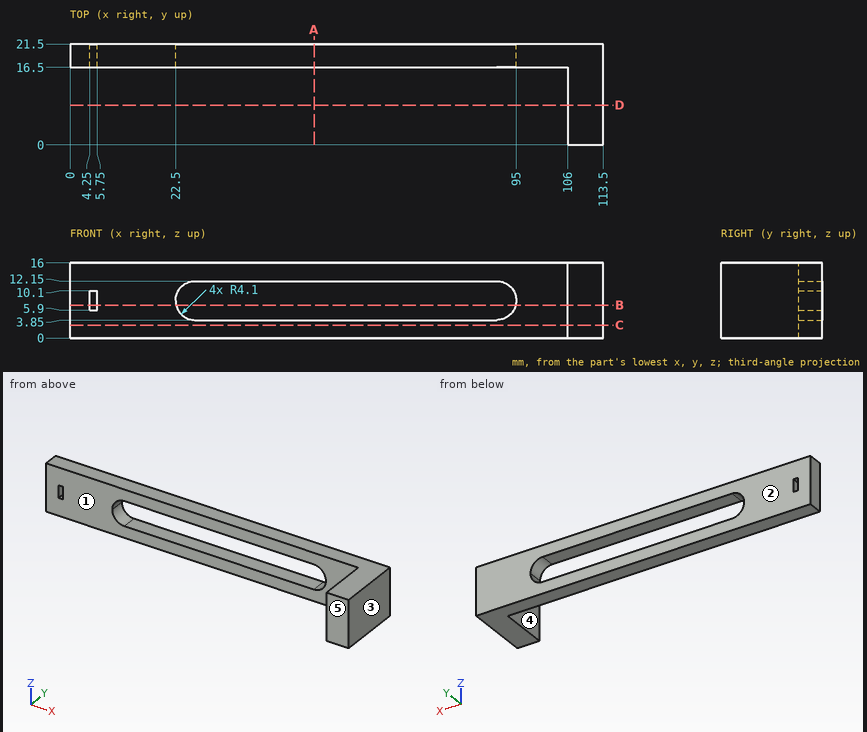
Design review of the part shown in the three views and the two pictorial views. Dimensions are in mm from the part's minimum x, y and z. A direction names the side the tool comes from. Give positions to 0.01 mm unless a question says otherwise; leave off trailing zeros. Loops run counter-clockwise (first coordinate to the right, second up) from the corner with the lowest first, then second, coordinate; pieces in that order, holes last. Notation, with made-up numbers: M -27,77 L 2,77 A30 cw 2,101 Z; hole C -13.75,70.25 d9. An arc over 180 degrees is marked long. Put each result on its own line as item: value. Start each with the question number.
(1) Machinability: for the marked faces 4 and 5, which of the approach directions +Z, -Z, +X, -X, +Y, -Y give a long, thin tool a straight path to every point of the face, cutting with its end or side? Answer none if there is none.
(2) Add section D-D, the plane y = 8.5. Write out the cut boundary in (x, z), then the cut area to 3 significant figures.
(3) Wall thickness on L1, parallel to X at y = 17.25, z = 7; L2, parallel to Y at x = 33.5, z = 12.5; L3, parallel to X at y = 9, z = 5.5: over which ranges is each line inside the solid? List them lowest first.
(4) Add section B-B, the plane z = 7. Write out the cut boundary in (x, y).
(5) For pin 1 (8 mm diameter, centred on y = 5, z = 7.5, fed in from -X); pin 2 (1.5 mm diameter, centred on x = 33.5, z = 12, fed in from -Y); pin 3 (4 mm diameter, centred on x = 66.5, y = 14, fed in from +Z), all flat-tipped, find the tip position at first contact; note any pin that passes through.
(6) Add section A-A, the plane x = 52. Write out the cut boundary in (y, z), then the cut area to 3 significant figures.
(7) Add section C-C, the plane z = 2.75. Write out the cut boundary in (x, y).
(8) The part is to be moulded in two halves that separate along Y. For the marked faces 1, 2 and 3, say which applies: +Y half, -Y half, draft (parallel to the pull), parting line (faces both ways), or undercut.
Result:
1. face 4: +Z, -Z, -X, -Y
1. face 5: +Z, -Z, +X, -X, -Y
2. outline: M 106,0 L 113.5,0 L 113.5,16 L 106,16 Z
2. area: 120 mm^2
3. L1: x = 0 to 4.25, 5.75 to 22.61, 94.89 to 113.5
3. L2: y = 16.5 to 21.5
3. L3: x = 106 to 113.5
4. outline: M 0,16.5 L 4.25,16.5 L 4.25,21.5 L 0,21.5 Z; M 5.75,16.5 L 22.61,16.5 L 22.61,21.5 L 5.75,21.5 Z; M 94.89,16.5 L 106,16.5 L 106,0 L 113.5,0 L 113.5,21.5 L 94.89,21.5 Z
5. pin 1: stops at x = 106
5. pin 2: stops at y = 16.5
5. pin 3: passes through
6. outline: M 16.5,0 L 21.5,0 L 21.5,3.85 L 16.5,3.85 Z; M 16.5,12.15 L 21.5,12.15 L 21.5,16 L 16.5,16 Z
6. area: 38.5 mm^2
7. outline: M 0,16.5 L 106,16.5 L 106,0 L 113.5,0 L 113.5,21.5 L 0,21.5 Z
8. face 1: -Y half
8. face 2: +Y half
8. face 3: draft
